Source: CAD feature listing. Evaluate the final solid. Frame: model axes, mm. Face numbers are marked on the shaded views. A direction names the side the tool comes from. Round coordinates to 2 decimals unless told otherwise and drop trailing zeros. Write each loop counter-clockwise with the first axis right and the second up, starting at its lowest first coordinate (ties: lowest second). Pieces come first, ordered by that corner, then holes.
from build123d import *

# Parameters (mm, degrees)
SKETCH1_W           = 3.7
SKETCH1_H           = 0.65
BOSS_EXTRUDE1_DEPTH = 6.5
SKETCH2_W           = 3.7
SKETCH2_H           = 0.65
BOSS_EXTRUDE2_DEPTH = 18
SKETCH5_W           = 6
SKETCH5_H           = 7.371976581
BOSS_EXTRUDE4_DEPTH = 10.3
BOSS_EXTRUDE4_TAPER = 5
SKETCH7_W           = 2.169554373
SKETCH7_H           = 1.15
CUT_EXTRUDE1_DEPTH  = 10.3
SKETCH9_W           = 1.15
SKETCH9_H           = 1.6
CUT_EXTRUDE2_DEPTH  = 10.3
SKETCH3_R           = 2
BOSS_EXTRUDE3_DEPTH = 20


with BuildPart() as part:
    # Sketch1 → Boss-Extrude1 (new body)
    with BuildSketch(Plane.XY):
        Polygon((1, 1.8), (0, 1), (0, 0), (6.8, 0), (6.8, 1), (5.8, 1.8), align=None)
        with Locations((3.4, 0.525)):
            Rectangle(SKETCH1_W, SKETCH1_H, mode=Mode.SUBTRACT)
    extrude(amount=BOSS_EXTRUDE1_DEPTH)

    # Sketch2 → Boss-Extrude2 (add)
    with BuildSketch(Plane.XY.offset(6.5)):
        Polygon((6.5, 4.8), (0.3, 4.8), (-1.9, 2.6), (-1.9, -3), (8.7, -3), (8.7, 2.6), align=None)
        Polygon((5.8, 1.8), (6.8, 1), (6.8, 0), (0, 0), (0, 1), (1, 1.8), align=None, mode=Mode.SUBTRACT)
        Polygon((6.8, 0), (6.8, 1), (5.8, 1.8), (1, 1.8), (0, 1), (0, 0), align=None)
        with Locations((3.4, 0.525)):
            Rectangle(SKETCH2_W, SKETCH2_H, mode=Mode.SUBTRACT)
        with Locations((3.4, 0.525)):
            Rectangle(SKETCH2_W, SKETCH2_H)
    extrude(amount=BOSS_EXTRUDE2_DEPTH)

    # Sketch5 → Boss-Extrude4 (add)
    with BuildSketch(Plane.XY.offset(24.5)):
        with Locations((3.4, 0.91401171)):
            Rectangle(SKETCH5_W, SKETCH5_H)
    extrude(amount=BOSS_EXTRUDE4_DEPTH, taper=BOSS_EXTRUDE4_TAPER)

    # Sketch7 → Cut-Extrude1 (cut)
    with BuildSketch(Plane(origin=(0, 4.8, 0), x_dir=(1, 0, 0), z_dir=(0, 1, 0))):
        Polygon((1.9, -25.65), (0.3, -25.65), (-0.269554373, -25.65), (-0.269554373, -26.8), (1.9, -26.8), align=None)
        with Locations((0.815222814, -28.525)):
            Rectangle(SKETCH7_W, SKETCH7_H)
        with Locations((0.815222814, -30.825)):
            Rectangle(SKETCH7_W, SKETCH7_H)
        with Locations((0.815222814, -33.125)):
            Rectangle(SKETCH7_W, SKETCH7_H)
        with Locations((5.984777187, -26.225)):
            Rectangle(SKETCH7_W, SKETCH7_H)
        with Locations((5.984777187, -28.525)):
            Rectangle(SKETCH7_W, SKETCH7_H)
        with Locations((5.984777187, -30.825)):
            Rectangle(SKETCH7_W, SKETCH7_H)
        with Locations((5.984777187, -33.125)):
            Rectangle(SKETCH7_W, SKETCH7_H)
    extrude(amount=-CUT_EXTRUDE1_DEPTH, mode=Mode.SUBTRACT)

    # Sketch9 → Cut-Extrude2 (cut)
    with BuildSketch(Plane(origin=(8.7, 0, 0), x_dir=(0, 0, -1), z_dir=(1, 0, 0))):
        with Locations((-26.225, 3.8)):
            Rectangle(SKETCH9_W, SKETCH9_H)
        with Locations((-30.825, 3.8)):
            Rectangle(SKETCH9_W, SKETCH9_H)
        with Locations((-26.225, -2)):
            Rectangle(SKETCH9_W, SKETCH9_H)
        with Locations((-30.825, -2)):
            Rectangle(SKETCH9_W, SKETCH9_H)
    extrude(amount=-CUT_EXTRUDE2_DEPTH, mode=Mode.SUBTRACT)

    # Sketch3 → Boss-Extrude3 (add)
    with BuildSketch(Plane.XY.offset(24.5)):
        with Locations((3.4, 0.9)):
            Circle(SKETCH3_R)
    extrude(amount=BOSS_EXTRUDE3_DEPTH)


solid = part.part
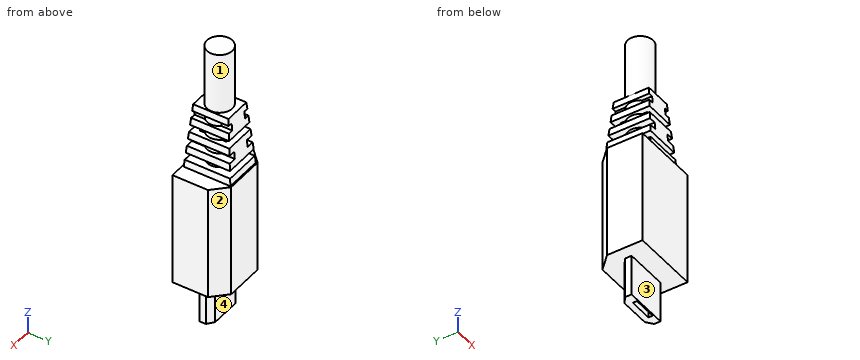
1) Material intervals for line 1 (Y direction, x = 5, z = 3); line 2 (Z direction, x = 5.25, y = 2.5); line 3 (Z direction, x = 0, y = 2.5), sorted ascending.
Taken from the geometry:
line 1: y = 0 to 0.2, 0.85 to 1.8
line 2: z = 6.5 to 25.65, 26.8 to 27.95, 29.1 to 30.25, 31.4 to 32.55, 33.7 to 34.8
line 3: z = 6.5 to 24.5
2) Section query A-A on z = 3. Return the cut outline in (x, y).
Taken from the geometry:
outline: (0, 0) - (6.8, 0) - (6.8, 1) - (5.8, 1.8) - (1, 1.8) - (0, 1) - close; hole (1.55, 0.2) - (5.25, 0.2) - (5.25, 0.85) - (1.55, 0.85) - close
3) Reachability of the marked faces 1, 2, 3 and 4 from +Z, -Z, +X, -X, +Y, -Y: full face, straight path, thin tool, end or side. Return the list, or none.
Taken from the geometry:
face 1: +Z
face 2: +Z, -Z, +X, +Y
face 3: -Z, +X, -X, -Y
face 4: -Z, +X, -X, +Y
4) Section query C-C on z = 42. Return the cut outline in (x, y), then the cut area to 3 significant figures.
Taken from the geometry:
outline: circle Ø4 at (3.4, 0.9)
area: 12.6 mm2
5) Contact query for flat-ended pins moving along their axis: P1, Ø2.5, axis at x = 3.5, z = 4, coming from the +Y side; P2, Ø0.8, axis at y = 0.5, z = 2.5, coming from the +X side; P3, Ø0.5, axis at y = 0.5, z = 2.5, coming from the -X side. Output: stop coordinate, or through.
Taken from the geometry:
P1: stops at y = 1.8
P2: stops at x = 6.8
P3: stops at x = 0
6) Section query B-B on z = 20.5. Return the cut outline in (x, y).
Taken from the geometry:
outline: (-1.9, -3) - (8.7, -3) - (8.7, 2.6) - (6.5, 4.8) - (0.3, 4.8) - (-1.9, 2.6) - close
